Input: part model. Units: mm. Frame: model coordinates. A direction names the side the tool comes from. Round coordinates to 2 decimals unless told otherwise and drop trailing zeros. Loops run counter-clockwise (first coordinate to the right, second up) from the corner with the lowest first, then second, coordinate; pieces in that order, holes last. Notation, with made-up numbers: (14, 63) -> (44, 63) arc R29 ccw to (44, 86) -> close; hole circle Ø5 at (-11, -36). An arc over 180 degrees is marked (long way). Answer as a JSON object with one key per item and string values. Group by question number.
Item 1: Section query C-C on x = 3. Return loops of the section in (y, z), and give its area (3 significant figures).
Item 2: Section query A-A on z = 0. Count the separate pieces of the cut face and the enclosed holes in it, and give its area (3 significant figures).
Item 3: Section query B-B on x = 13.5. Return loops of the section in (y, z).
Item 4: Material intervals for line 1 (Y direction, x = 36.5, z = 0.5); line 2 (Z direction, x = 13.5, y = -0.7); line 3 (X direction, y = 57, z = 11.75), sorted ascending. Write a range as [from, to].
Item 5: Draft query along Y for faces 1 (the flat face through (35, 35, 0)), 2 (the flat face through (0, 21.36, -12)), 3 (the cylindrical face through (-37.47, 55.7, 4.87)). Return one class per face: released by +Y, released by -Y, zero draft, split by the parting line, or undercut.
Item 6: Set-up query: faces 4 (the flat face through (40, 32, 0)), 5 (the flat face through (0, 12, -10)), 6 (the flat face through (-35, 35, 0)). Return all of +Z, -Z, +X, -X, +Y, -Y with unobstructed straight access to the full face (end or side cutting, diameter ignored); none if empty.
Item 7: Pin query (flat end, axial travel): pin 1 (9 mm diameter, centred on y = 29.5, z = 3.5, fed in from -X); pin 2 (5.5 mm diameter, centred on x = 3, y = 16, fed in from +Z); pin 3 (4 mm diameter, centred on x = -1, z = -13.5, fed in from +Y); pin 4 (1.5 mm diameter, centred on x = 7, z = 12, fed in from +Y). Return the tip coordinate at first contact, or that it passes through.
from build123d import *

# Parameters (mm, degrees)
F0_W     = 5
F0_H     = 65
F1_DEPTH = 15
F2_R     = 8
F3_DEPTH = 12.5
F6_DEPTH = 50
F9_START = -10
F8_W     = 20
F8_H     = 20
F9_DEPTH = 5


with BuildPart() as f1:
    # F0 (on Top) → F1 (new body, symmetric)
    with BuildSketch(Plane.XY):
        Polygon((40, -2.5), (40, 2.5), (35, 2.5), (-35, 2.5), (-40, 2.5), (-40, -2.5), align=None)
        with Locations((37.5, 35)):
            Rectangle(F0_W, F0_H)
        with Locations((-37.5, 35)):
            Rectangle(F0_W, F0_H)
    extrude(amount=F1_DEPTH, both=True)


with BuildPart() as f3:
    # F2 (on Front) → F3 (new body, symmetric)
    with BuildSketch(Plane.XZ):
        with Locations((-13.5, 0)):
            Circle(F2_R)
    extrude(amount=F3_DEPTH, both=True)


with BuildPart() as f3b:
    # F2 (on Front) → F3, piece 2 (new body, symmetric)
    with BuildSketch(Plane.XZ):
        with BuildLine():
            ThreePointArc((21.5, 0), (13.5, 8), (5.5, 0))
            ThreePointArc((5.5, 0), (13.5, -8), (21.5, 0))
        make_face()
    extrude(amount=F3_DEPTH, both=True)


with BuildPart() as f1_1:
    add(f1.part)

    # F4: cut F3, F3b
    add(f3.part, mode=Mode.SUBTRACT)
    add(f3b.part, mode=Mode.SUBTRACT)


with BuildPart() as f6:
    # F5 (on Right) → F6 (new body, symmetric)
    with BuildSketch(Plane.YZ):
        with BuildLine():
            Line((22.3510495666, 0), (30.3510495666, 0))
            ThreePointArc((30.3510495666, 0), (22.3510495666, 8), (14.3510495666, 0))
            Line((14.3510495666, 0), (22.3510495666, 0))
        make_face()
        with BuildLine():
            ThreePointArc((14.3510495666, 0), (22.3510495666, -8), (30.3510495666, 0))
            Line((30.3510495666, 0), (22.3510495666, 0))
            Line((22.3510495666, 0), (14.3510495666, 0))
        make_face()
    extrude(amount=F6_DEPTH, both=True)


with BuildPart() as f6b:
    # F5 (on Right) → F6, piece 2 (new body, symmetric)
    with BuildSketch(Plane.YZ):
        with BuildLine():
            ThreePointArc((57.3510495666, 0), (49.3510495666, 8), (41.3510495666, 0))
            ThreePointArc((41.3510495666, 0), (49.3510495666, -8), (57.3510495666, 0))
        make_face()
    extrude(amount=F6_DEPTH, both=True)


with BuildPart() as f1_2:
    add(f1_1.part)

    # F7: cut F6, F6b
    add(f6.part, mode=Mode.SUBTRACT)
    add(f6b.part, mode=Mode.SUBTRACT)

    # F8 (on Top) → F9 (join)
    with BuildSketch(Plane.XY.offset(F9_START)):
        with Locations((-0.1337498054, 11.3596525043)):
            Rectangle(F8_W, F8_H)
    extrude(amount=-F9_DEPTH)


solid = f1_2.part
Solved:
{
 "1": {"outline": "(-2.5, -15) -> (21.36, -15) -> (21.36, -10) -> (2.5, -10) -> (2.5, 15) -> (-2.5, 15) -> close", "area": "244 mm²"},
 "2": {"separate pieces": "7", "enclosed holes": "0", "area": "570 mm²"},
 "3": {"outline": "(-2.5, -15) -> (2.5, -15) -> (2.5, -8) -> (-2.5, -8) -> close; (-2.5, 8) -> (2.5, 8) -> (2.5, 15) -> (-2.5, 15) -> close"},
 "4": {"line 1": "[-2.5, 14.37], [30.34, 41.37], [57.34, 67.5]", "line 2": "[-15, -8], [8, 15]", "line 3": "[-40, -35], [35, 40]"},
 "5": {"face 1": "zero draft", "face 2": "released by +Y", "face 3": "undercut"},
 "6": {"face 4": "+Z, -Z, +X, +Y, -Y", "face 5": "+Z, +Y", "face 6": "+Z, -Z, +Y"},
 "7": {"pin 1": "x = -40", "pin 2": "z = -10", "pin 3": "y = 21.36", "pin 4": "y = 2.5"}
}
